Could you check a few things on this drawing? It's one solid part, dimensions in mm from its lowest x, y, z. Coordinates: 2 decimals unless noted, no trailing zeros. Loops run counter-clockwise (first coordinate to the right, second up) from the corner with the lowest first, then second, coordinate; pieces in that order, holes last. Notation, with made-up numbers: (-5, 72.25) -> (54, 72.25) arc R9 cw to (54, 89.25) -> close; hole circle Ø9 at (50.25, 0.5). An arc over 180 degrees is marked (long way). One line per question, with ' | ' between items. Start each with the question number.
(1) Suppose I cut it at A-A (y = 4.75). Please give me the cut outline in (x, z), plus the area to 3 significant figures.
(2) Suppose I cut it at C-C (z = 0.45). Please give me the cut outline in (x, y), plus the area to 3 significant figures.
(3) Suppose I cut it at B-B (z = 2.75). Please give me the cut outline in (x, y), plus the area to 3 significant figures.
(4) If I drill on line 1 along X through (y, z) = (16.75, 0.9); line 2 along X through (y, z) = (12.75, 2.75); line 3 along Z through (x, y) = (12.25, 4), over which ranges is the centre line in solid material (lowest first)?
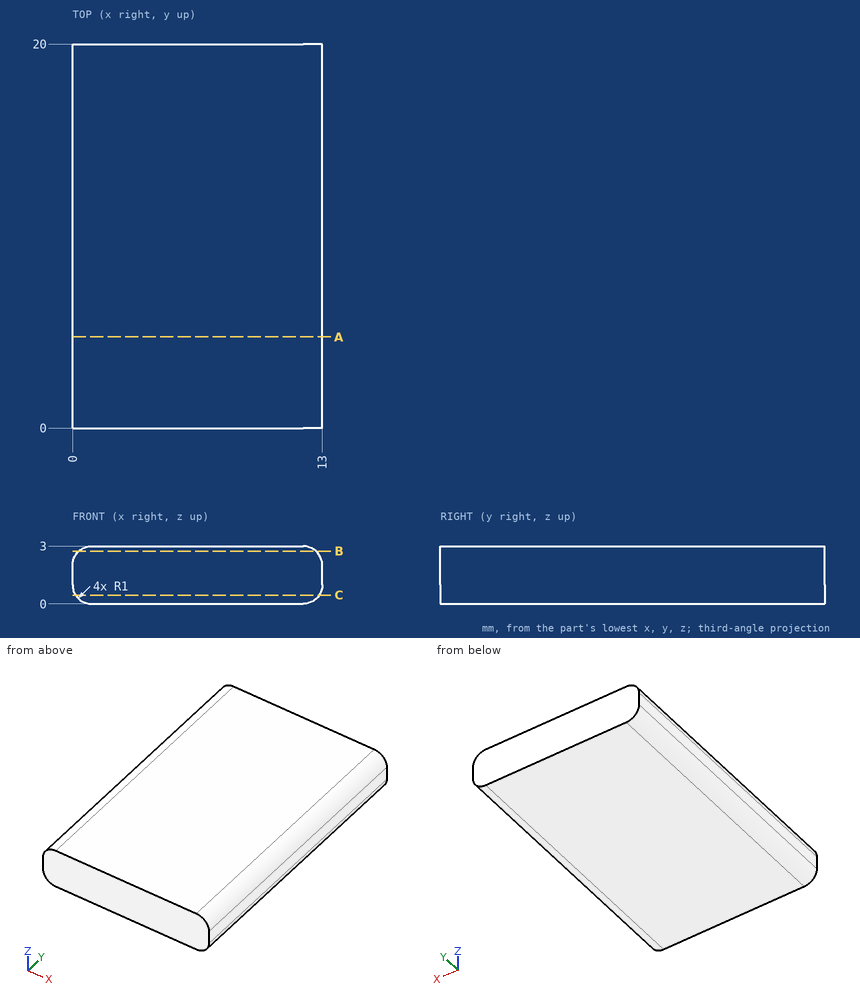
Checks:
1) outline: (0, 1) arc R1 ccw to (1, 0) -> (12, 0) arc R1 ccw to (13, 1) -> (13, 2) arc R1 ccw to (12, 3) -> (1, 3) arc R1 ccw to (0, 2) -> close | area: 38.1 mm^2
2) outline: (0.16, 0) -> (12.84, 0) -> (12.84, 20) -> (0.16, 20) -> close | area: 253 mm^2
3) outline: (0.34, 0) -> (12.66, 0) -> (12.66, 20) -> (0.34, 20) -> close | area: 246 mm^2
4) line 1: x = 0.01 to 12.99 | line 2: x = 0.34 to 12.66 | line 3: z = 0.03 to 2.97
